Verification items for the finished model (mm, model axes). A direction names the side the tool comes from. Give positions to 0.01 mm unless a question says otherwise; leave off trailing zeros. Write each loop counter-clockwise with the first axis right and the second up, starting at its lowest first coordinate (ties: lowest second). Pieces come first, ordered by that corner, then holes. Notation, with made-up numbers: (2.5, 14) -> (50.5, 14) arc R23 cw to (50.5, 49) -> close; hole circle Ø7 at (84, -40). An arc over 180 degrees is marked (long way). Answer as CSV lines item,"result". Start each with the question number.
1) Material ranges on L1, parallel to Y at x = -11.7, z = -27.5; L2, parallel to Y at x = 5, z = -20 (3 decimals); L3, parallel to X at y = -10.5, z = -42.5, recorded low to high.
2) Sectioned sample at C-C on y = 0. Record the cut outline in (x, z), and give its area (3 significant figures).
3) Tool access check on faces 3 (the flat face through (15, 9, -11)), 4 (the flat face through (11, 8.25, -11)). Record the directions out of +Z, -Z, +X, -X, +Y, -Y that give a thin tool (end or side, any length) a straight path to the whole face; none if there is none.
4) Gauge pin test, flat ends, axial feed: pin 1 Ø3.5 at (x, y) = (11.7, -11.7) entering from -Z; pin 2 Ø1 at (y, z) = (-1.5, -10.5) entering from +X; pin 3 Ø7 at (x, z) = (-1, -28) entering from +Y. Record the tip position at first contact, or that the pin passes through.
5) Sectioned sample at A-A on y = -11.7. Record the cut outline in (x, z).
6) Mould release check, pull along Y, two halves, no side actions. Record for faces 1 (the flat face through (-4, 0, 30)), 2 (the flat face through (-5.8, 0, -11)): released by +Y, released by -Y, zero draft, split by the parting line, or undercut.
```python
from build123d import *

# Parameters (mm, degrees)
CROQUIS1_R              = 2.1
CROQUIS1_R_2            = 3.4
SALIENTE_EXTRUIR1_DEPTH = 400
CROQUIS2_W              = 38.422022472
CROQUIS2_H              = 31.615605493
CORTAR_EXTRUIR1_DEPTH   = 320


with BuildPart() as part:
    # Croquis1 → Saliente-Extruir1 (new body)
    with BuildSketch(Plane(origin=(0, 0, -50), x_dir=(-1, 0, 0), z_dir=(0, 0, -1))):
        with BuildLine():
            Line((14.7, -5.1), (14.3, -5.1))
            ThreePointArc((14.3, -5.1), (14.087867966, -5.012132034), (14, -4.8))
            Line((14, -4.8), (14, -4.4))
            ThreePointArc((14, -4.4), (13.912132034, -4.187867966), (13.7, -4.1))
            Line((13.7, -4.1), (13.3, -4.1))
            ThreePointArc((13.3, -4.1), (13.087867966, -4.187867966), (13, -4.4))
            Line((13, -4.4), (13, -7.95))
            ThreePointArc((13, -7.95), (12.912132034, -8.162132034), (12.7, -8.25))
            Line((12.7, -8.25), (9.789264108, -8.25))
            ThreePointArc((9.789264108, -8.25), (9.674477865, -8.22717164), (9.577160832, -8.162160788))
            Line((9.577160832, -8.162160788), (5.887896723, -4.473896751))
            ThreePointArc((5.887896723, -4.473896751), (5.822843922, -4.376559778), (5.8, -4.261735963))
            Line((5.8, -4.261735963), (5.8, 4.260735931))
            ThreePointArc((5.8, 4.260735931), (5.82283614, 4.375540961), (5.887867966, 4.472867966))
            Line((5.887867966, 4.472867966), (9.577132034, 8.162132034))
            ThreePointArc((9.577132034, 8.162132034), (9.674459039, 8.22716386), (9.789264069, 8.25))
            Line((9.789264069, 8.25), (12.7, 8.25))
            ThreePointArc((12.7, 8.25), (12.912132034, 8.162132034), (13, 7.95))
            Line((13, 7.95), (13, 4.4))
            ThreePointArc((13, 4.4), (13.087867966, 4.187867966), (13.3, 4.1))
            Line((13.3, 4.1), (13.7, 4.1))
            ThreePointArc((13.7, 4.1), (13.912132034, 4.187867966), (14, 4.4))
            Line((14, 4.4), (14, 4.8))
            ThreePointArc((14, 4.8), (14.087867966, 5.012132034), (14.3, 5.1))
            Line((14.3, 5.1), (14.7, 5.1))
            ThreePointArc((14.7, 5.1), (14.912132034, 5.187867966), (15, 5.4))
            Line((15, 5.4), (15, 12.5))
            ThreePointArc((15, 12.5), (14.267766953, 14.267766953), (12.5, 15))
            Line((12.5, 15), (5.4, 15))
            ThreePointArc((5.4, 15), (5.187867966, 14.912132034), (5.1, 14.7))
            Line((5.1, 14.7), (5.1, 14.3))
            ThreePointArc((5.1, 14.3), (5.012132034, 14.087867966), (4.8, 14))
            Line((4.8, 14), (4.4, 14))
            ThreePointArc((4.4, 14), (4.187867966, 13.912132034), (4.1, 13.7))
            Line((4.1, 13.7), (4.1, 13.3))
            ThreePointArc((4.1, 13.3), (4.187867966, 13.087867966), (4.4, 13))
            Line((4.4, 13), (7.95, 13))
            ThreePointArc((7.95, 13), (8.162132034, 12.912132034), (8.25, 12.7))
            Line((8.25, 12.7), (8.25, 9.788264069))
            ThreePointArc((8.25, 9.788264069), (8.22716386, 9.673459039), (8.162132034, 9.576132034))
            Line((8.162132034, 9.576132034), (4.473867966, 5.887867966))
            ThreePointArc((4.473867966, 5.887867966), (4.376540961, 5.82283614), (4.261735931, 5.8))
            Line((4.261735931, 5.8), (-4.260735892, 5.8))
            ThreePointArc((-4.260735892, 5.8), (-4.375522135, 5.82282836), (-4.472839168, 5.887839212))
            Line((-4.472839168, 5.887839212), (-8.162103277, 9.576103249))
            ThreePointArc((-8.162103277, 9.576103249), (-8.227156078, 9.673440222), (-8.25, 9.788264037))
            Line((-8.25, 9.788264037), (-8.25, 12.7))
            ThreePointArc((-8.25, 12.7), (-8.162132034, 12.912132034), (-7.95, 13))
            Line((-7.95, 13), (-4.4, 13))
            ThreePointArc((-4.4, 13), (-4.187867966, 13.087867966), (-4.1, 13.3))
            Line((-4.1, 13.3), (-4.1, 13.7))
            ThreePointArc((-4.1, 13.7), (-4.187867966, 13.912132034), (-4.4, 14))
            Line((-4.4, 14), (-4.8, 14))
            ThreePointArc((-4.8, 14), (-5.012132034, 14.087867966), (-5.1, 14.3))
            Line((-5.1, 14.3), (-5.1, 14.7))
            ThreePointArc((-5.1, 14.7), (-5.187867966, 14.912132034), (-5.4, 15))
            Line((-5.4, 15), (-12.5, 15))
            ThreePointArc((-12.5, 15), (-14.267766953, 14.267766953), (-15, 12.5))
            Line((-15, 12.5), (-15, 5.4))
            ThreePointArc((-15, 5.4), (-14.912132034, 5.187867966), (-14.7, 5.1))
            Line((-14.7, 5.1), (-14.3, 5.1))
            ThreePointArc((-14.3, 5.1), (-14.087867966, 5.012132034), (-14, 4.8))
            Line((-14, 4.8), (-14, 4.4))
            ThreePointArc((-14, 4.4), (-13.912132034, 4.187867966), (-13.7, 4.1))
            Line((-13.7, 4.1), (-13.3, 4.1))
            ThreePointArc((-13.3, 4.1), (-13.087867966, 4.187867966), (-13, 4.4))
            Line((-13, 4.4), (-13, 7.95))
            ThreePointArc((-13, 7.95), (-12.912132034, 8.162132034), (-12.7, 8.25))
            Line((-12.7, 8.25), (-9.788264037, 8.25))
            ThreePointArc((-9.788264037, 8.25), (-9.673440222, 8.227156078), (-9.576103249, 8.162103277))
            Line((-9.576103249, 8.162103277), (-5.887839212, 4.472839168))
            ThreePointArc((-5.887839212, 4.472839168), (-5.82282836, 4.375522135), (-5.8, 4.260735892))
            Line((-5.8, 4.260735892), (-5.8, -4.261735931))
            ThreePointArc((-5.8, -4.261735931), (-5.82283614, -4.376540961), (-5.887867966, -4.473867966))
            Line((-5.887867966, -4.473867966), (-9.576132034, -8.162132034))
            ThreePointArc((-9.576132034, -8.162132034), (-9.673459039, -8.22716386), (-9.788264069, -8.25))
            Line((-9.788264069, -8.25), (-12.7, -8.25))
            ThreePointArc((-12.7, -8.25), (-12.912132034, -8.162132034), (-13, -7.95))
            Line((-13, -7.95), (-13, -4.4))
            ThreePointArc((-13, -4.4), (-13.087867966, -4.187867966), (-13.3, -4.1))
            Line((-13.3, -4.1), (-13.7, -4.1))
            ThreePointArc((-13.7, -4.1), (-13.912132034, -4.187867966), (-14, -4.4))
            Line((-14, -4.4), (-14, -4.8))
            ThreePointArc((-14, -4.8), (-14.087867966, -5.012132034), (-14.3, -5.1))
            Line((-14.3, -5.1), (-14.7, -5.1))
            ThreePointArc((-14.7, -5.1), (-14.912132034, -5.187867966), (-15, -5.4))
            Line((-15, -5.4), (-15, -12.5))
            ThreePointArc((-15, -12.5), (-14.267766953, -14.267766953), (-12.5, -15))
            Line((-12.5, -15), (-5.4, -15))
            ThreePointArc((-5.4, -15), (-5.187867966, -14.912132034), (-5.1, -14.7))
            Line((-5.1, -14.7), (-5.1, -14.3))
            ThreePointArc((-5.1, -14.3), (-5.012132034, -14.087867966), (-4.8, -14))
            Line((-4.8, -14), (-4.4, -14))
            ThreePointArc((-4.4, -14), (-4.187867966, -13.912132034), (-4.1, -13.7))
            Line((-4.1, -13.7), (-4.1, -13.3))
            ThreePointArc((-4.1, -13.3), (-4.187867966, -13.087867966), (-4.4, -13))
            Line((-4.4, -13), (-7.95, -13))
            ThreePointArc((-7.95, -13), (-8.162132034, -12.912132034), (-8.25, -12.7))
            Line((-8.25, -12.7), (-8.25, -9.789264069))
            ThreePointArc((-8.25, -9.789264069), (-8.22716386, -9.674459039), (-8.162132034, -9.577132034))
            Line((-8.162132034, -9.577132034), (-4.472867966, -5.887867966))
            ThreePointArc((-4.472867966, -5.887867966), (-4.375540961, -5.82283614), (-4.260735931, -5.8))
            Line((-4.260735931, -5.8), (4.261735963, -5.8))
            ThreePointArc((4.261735963, -5.8), (4.376559778, -5.822843922), (4.473896751, -5.887896723))
            Line((4.473896751, -5.887896723), (8.162160788, -9.577160832))
            ThreePointArc((8.162160788, -9.577160832), (8.22717164, -9.674477865), (8.25, -9.789264108))
            Line((8.25, -9.789264108), (8.25, -12.7))
            ThreePointArc((8.25, -12.7), (8.162132034, -12.912132034), (7.95, -13))
            Line((7.95, -13), (4.4, -13))
            ThreePointArc((4.4, -13), (4.187867966, -13.087867966), (4.1, -13.3))
            Line((4.1, -13.3), (4.1, -13.7))
            ThreePointArc((4.1, -13.7), (4.187867966, -13.912132034), (4.4, -14))
            Line((4.4, -14), (4.8, -14))
            ThreePointArc((4.8, -14), (5.012132034, -14.087867966), (5.1, -14.3))
            Line((5.1, -14.3), (5.1, -14.7))
            ThreePointArc((5.1, -14.7), (5.187867966, -14.912132034), (5.4, -15))
            Line((5.4, -15), (12.5, -15))
            ThreePointArc((12.5, -15), (14.267766953, -14.267766953), (15, -12.5))
            Line((15, -12.5), (15, -5.4))
            ThreePointArc((15, -5.4), (14.912132034, -5.187867966), (14.7, -5.1))
        make_face()
        with Locations((-11.7, 11.7)):
            Circle(CROQUIS1_R, mode=Mode.SUBTRACT)
        with Locations((-11.7, -11.7)):
            Circle(CROQUIS1_R, mode=Mode.SUBTRACT)
        Circle(CROQUIS1_R_2, mode=Mode.SUBTRACT)
        with Locations((11.7, 11.7)):
            Circle(CROQUIS1_R, mode=Mode.SUBTRACT)
        with Locations((11.7, -11.7)):
            Circle(CROQUIS1_R, mode=Mode.SUBTRACT)
    extrude(amount=-SALIENTE_EXTRUIR1_DEPTH)

    # Croquis2 → Cortar-Extruir1 (cut)
    with BuildSketch(Plane.XY.offset(350)):
        with Locations((1.308926342, 0.261785268)):
            Rectangle(CROQUIS2_W, CROQUIS2_H)
    extrude(amount=-CORTAR_EXTRUIR1_DEPTH, mode=Mode.SUBTRACT)


solid = part.part
```
Ans:
1,L1,"y = -15 to -13.8, -9.6 to -8.25, 8.25 to 9.6, 13.8 to 15"
1,L2,"y = -14.076 to -13, -6.415 to 6.415, 13 to 14.076"
1,L3,"x = -15 to -13.42, -9.98 to -8.25, 8.25 to 9.98, 13.42 to 15"
2,outline,"(-5.8, -50) -> (-3.4, -50) -> (-3.4, 30) -> (-5.8, 30) -> close; (3.4, -50) -> (5.8, -50) -> (5.8, 30) -> (3.4, 30) -> close"
2,area,"384 mm²"
3,face 3,"+Z, -Z, +X, +Y, -Y"
3,face 4,"+Z, -Z"
4,pin 1,"passes through"
4,pin 2,"stops at x = 5.8"
4,pin 3,"stops at y = 14"
5,outline,"(-15, -50) -> (-13.8, -50) -> (-13.8, 30) -> (-15, 30) -> close; (-9.6, -50) -> (-8.25, -50) -> (-8.25, 30) -> (-9.6, 30) -> close; (8.25, -50) -> (9.6, -50) -> (9.6, 30) -> (8.25, 30) -> close; (13.8, -50) -> (15, -50) -> (15, 30) -> (13.8, 30) -> close"
6,face 1,"zero draft"
6,face 2,"undercut"
